Can you work these out from the model? Positions are in its coordinate system, mm. Face numbers are marked on the shaded views. A direction names the side the tool comes from. Round coordinates to 2 decimals unless told otherwise and drop trailing zeros. Loops run counter-clockwise (first coordinate to the right, second up) from the corner with the lowest first, then second, coordinate; pieces in that order, holes last. Notation, with made-up numbers: (78.25, 30.5) -> (89.25, 30.5) arc R19 cw to (89.25, 65.5) -> close; hole circle Ø5 at (87, 58.25). An arc over 180 degrees is marked (long way). Write item = value, one per line.
from build123d import *

# Parameters (mm, degrees)
AUFSATZ_LINEAR_AUSTRAGEN2_DEPTH = 18
SKIZZE3_W                       = 10.8
SKIZZE3_H                       = 4
SKIZZE3_H_2                     = 16
SKIZZE3_H_3                     = 8
SCHNITT_LINEAR_AUSTRAGEN1_DEPTH = 201.709049372
SCHNITT_LINEAR_AUSTRAGEN2_DEPTH = 203.940249827


with BuildPart() as part:
    # Skizze1 → Aufsatz-Linear austragen2 (new, symmetric)
    with BuildSketch(Plane.XY):
        with BuildLine():
            Line((-198.15, 0), (-198.15, -2))
            Line((-198.15, -2), (-199.65, -2))
            Line((-199.65, -2), (-199.65, 0))
            ThreePointArc((-199.65, 0), (-198.288046533, 3.288046533), (-195, 4.65))
            Line((-195, 4.65), (195, 4.65))
            ThreePointArc((195, 4.65), (198.288046533, 3.288046533), (199.65, 0))
            Line((199.65, 0), (199.65, -2))
            Line((199.65, -2), (198.15, -2))
            Line((198.15, -2), (198.15, 0))
            ThreePointArc((198.15, 0), (195, 3.15), (191.85, 0))
            Line((191.85, 0), (191.85, -2))
            Line((191.85, -2), (188.85, -2))
            Line((188.85, -2), (188.85, -5.35))
            Line((188.85, -5.35), (-188.85, -5.35))
            Line((-188.85, -5.35), (-188.85, -2))
            Line((-188.85, -2), (-191.85, -2))
            Line((-191.85, -2), (-191.85, 0))
            ThreePointArc((-191.85, 0), (-195, 3.15), (-198.15, 0))
        make_face()
    extrude(amount=AUFSATZ_LINEAR_AUSTRAGEN2_DEPTH, both=True)

    # Skizze3 → Schnitt-Linear austragen1 (cut, through all)
    with BuildSketch(Plane.XZ.offset(5.35)):
        with Locations((-194.25, 16)):
            Rectangle(SKIZZE3_W, SKIZZE3_H)
        with Locations((-194.25, 2)):
            Rectangle(SKIZZE3_W, SKIZZE3_H_2)
        with Locations((-194.25, -14)):
            Rectangle(SKIZZE3_W, SKIZZE3_H_3)
        with Locations((194.25, 14)):
            Rectangle(SKIZZE3_W, SKIZZE3_H_3)
        with Locations((194.25, -2)):
            Rectangle(SKIZZE3_W, SKIZZE3_H_2)
        with Locations((194.25, -16)):
            Rectangle(SKIZZE3_W, SKIZZE3_H)
    extrude(amount=-SCHNITT_LINEAR_AUSTRAGEN1_DEPTH, mode=Mode.SUBTRACT)

    # Skizze4 → Schnitt-Linear austragen2 (cut, through all)
    with BuildSketch(Plane.XY.offset(18)):
        Polygon((174.5, 4.65), (174.5, 3.15), (184.5, 3.15), (184.5, -5.35), (-199.65, -5.35), (-199.65, 4.65), align=None)
    extrude(amount=-SCHNITT_LINEAR_AUSTRAGEN2_DEPTH, mode=Mode.SUBTRACT)


solid = part.part
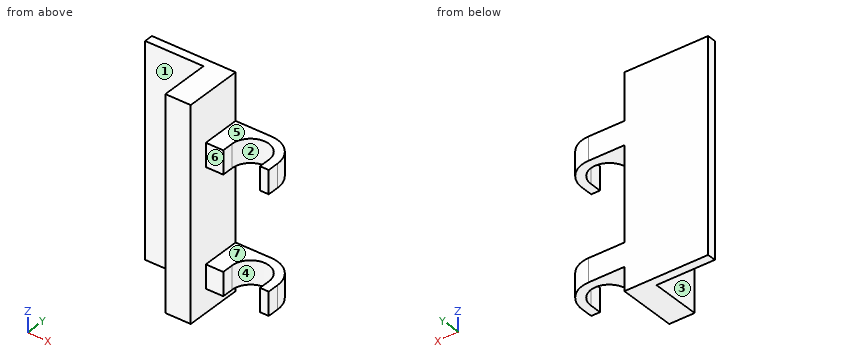
1. For the marked faces 4, 5, 6 and 7, which set-ups out of +Z, -Z, +X, -X, +Y, -Y let a thin tool reach every point of the face, with its end or its side?
Entries:
face_4 = +Z, -Z, -Y
face_5 = +Z, +X, +Y, -Y
face_6 = +Z, -Z, +X, -Y
face_7 = +X, +Y, -Y
2. Suppose I cut it at B-B, the plane z = 7.5. List the corners of the cut face in (x, y) for me.
Entries:
outline = (174.5, 3.15) -> (184.5, 3.15) -> (184.5, -5.35) -> (188.85, -5.35) -> (188.85, -2) -> (191.85, -2) -> (191.85, 0) arc R3.15 cw to (198.15, 0) -> (198.15, -2) -> (199.65, -2) -> (199.65, 0) arc R4.65 ccw to (195, 4.65) -> (174.5, 4.65) -> close
3. Suppose I cut it at A-A, the plane y = -1.5. List the corners of the cut face in (x, z) for me, and give its area (3 significant figures).
Entries:
outline = (184.5, -18) -> (188.85, -18) -> (188.85, -14) -> (191.85, -14) -> (191.85, -10) -> (188.85, -10) -> (188.85, 6) -> (191.85, 6) -> (191.85, 10) -> (188.85, 10) -> (188.85, 18) -> (184.5, 18) -> close; (198.15, -14) -> (199.65, -14) -> (199.65, -10) -> (198.15, -10) -> close; (198.15, 6) -> (199.65, 6) -> (199.65, 10) -> (198.15, 10) -> close
area = 193 mm²
4. Suppose I cut it at C-C, the plane x = 177.5. List the corners of the cut face in (y, z) for me, and give its area (3 significant figures).
Entries:
outline = (3.15, -18) -> (4.65, -18) -> (4.65, 18) -> (3.15, 18) -> close
area = 54.0 mm²
5. We'd pull the mould along X, two halves only. Please class the marked faces 1, 2 and 3: released by +X, released by -X, zero draft, split by the parting line, or undercut.
Entries:
face_1 = zero draft
face_2 = undercut
face_3 = released by -X
6. Suppose I cut it at D-D, the plane z = 15. List the corners of the cut face in (x, y) for me, and give its area (3 significant figures).
Entries:
outline = (174.5, 3.15) -> (184.5, 3.15) -> (184.5, -5.35) -> (188.85, -5.35) -> (188.85, 4.65) -> (174.5, 4.65) -> close
area = 58.5 mm²
7. I'm going to push flat-ended pins straight in: pin 1 (1.2 mm diameter, centred on x = 199.5, z = 9, fed in from -Y); pin 2 (0.6 mm diameter, centred on y = -1, z = 8.5, fed in from -X); pin 3 (3.5 mm diameter, centred on x = 196.5, y = 0, fed in from -Z); pin 4 (3.5 mm diameter, centred on x = 194.5, y = 1, fed in from -Z). Where does each tip first touch, or does it pass through?
Entries:
pin_1 = -2
pin_2 = 184.5
pin_3 = -14
pin_4 = through
8. I need wall thicknesses on line 1 (Z direction, x = 189.5, y = 0.75); line 2 (X direction, y = 3.25, z = -5); line 3 (X direction, y = 1.25, z = 5). Which ranges of each line are inside material? Lowest first, please. Write a range as [from, to].
Entries:
line_1 = [-14, -10], [6, 10]
line_2 = [174.5, 188.85]
line_3 = [184.5, 188.85]
